Autodesk Inventor part; units mm, degrees
ref_plane "Work Plane1" through (0, 0, 0) normal (0, 0, 1) x (1, 0, 0)
ref_plane "YZ Plane" through (0, 0, 0) normal (1, 0, 0) x (0, 1, 0)
ref_plane "XZ Plane" through (0, 0, 0) normal (0, 1, 0) x (-1, 0, 0)
ref_plane "Work Plane1" through (0, 0, 0) normal (0, 0, 1) x (1, 0, 0)
sketch "Sketch1" plane through (0, 0, 0) normal (0, 0, 1) x (1, 0, 0)
  line L0 (-155.0476, 232.0666) -> (-62.9335, 193.9117) construction
  line L1 (177.2752, 94.414) -> (270.7225, 55.7069) construction
  line L2 (177.2752, -94.414) -> (270.7225, -55.7069) construction
  line L3 (-155.0476, -232.0666) -> (-62.9335, -193.9117) construction
  line L4 (-192.4394, 0.4878) -> (-152.8157, 221.8622) construction
  line L5 (-152.8157, -221.8622) -> (-192.4394, -0.4878) construction
  line L6 (302.4733, 35) -> (302.4733, 38) construction
  line L7 (302.4733, -38) -> (302.4733, -35) construction
  line L8 (-254.8213, 5) -> (-254.8213, -5) construction
  line L9 (-272.5267, 75) -> (-179.1025, 75)
  line L10 (-179.1025, 75) -> (-179.1025, -75)
  line L11 (-179.1025, -75) -> (-272.5267, -75)
  line L12 (-272.5267, -75) -> (-272.5267, 75)
  line L13 (327.4733, 53.8478) -> (327.4733, 38) construction
  line L14 (-272.5267, 5) -> (-272.5267, -5) construction
  line L15 (327.4733, 42.5553) -> (302.4733, 42.5553)
  line L16 (302.4733, 42.5553) -> (302.4733, -42.5553)
  line L17 (302.4733, -42.5553) -> (327.4733, -42.5553)
  line L18 (327.4733, -42.5553) -> (327.4733, 42.5553)
  line L19 (-155.0476, 232.0666) -> (302.4733, 42.5553)
  line L20 (-155.0476, -232.0666) -> (302.4733, -42.5553)
  line L21 (-155.0476, 232.0666) -> (-179.1025, 75)
  line L22 (-179.1025, -75) -> (-155.0476, -232.0666)
  point P0 (0, 0)
  point P1 (-151.2693, 230.5016)
  point P2 (-151.2693, -230.5016)
  dimension "d0" = 150
extrude "Extrusion1" add sketch "Sketch1" along normal blind 10
properties part number "internalSupportBottom1" material "Wood (Birch)"
Could you check a few things on this model? Use its own coordinates, in mm. Coordinates: 2 decimals unless noted, no trailing zeros. Loops run counter-clockwise (first coordinate to the right, second up) from the corner with the lowest first, then second, coordinate; pieces in that order, holes last.
1. I need wall thicknesses on L1, parallel to Y at x = -187.5, z = 0.75; L2, parallel to X at y = 60, z = 3; L3, parallel to Y at x = -125.5, z = 6.5. Which ranges of each line are inside material? Lowest first, please.
2. Imagine slicing it at A-A (z = 4.5). Please give me the cut outline in (x, y), and give its area (3 significant figures).
3. Imagine slicing it at B-B (x = -212). Please give me the cut outline in (y, z).
4. Imagine slicing it at C-C (y = -91.5). Please give me the cut outline in (x, z).
5. For P1, Ø5, axis at x = 121.5, z = 4, coming from the +Y side; P2, Ø1.5, axis at x = -151.5, z = 8.5, coming from the +Y side; P3, Ø4, axis at y = -70.5, z = 2.5, coming from the +X side; P4, Ø5, axis at x = 40.5, y = -154.5, coming from the +Z side, each with a flat end and sliding along its axis, tell me the tip position at first contact or that it passes through.
Computed values:
1. L1: y = -75 to 75
1. L2: x = -272.53 to 260.36
1. L3: y = -219.83 to 219.83
2. outline: (-272.53, -75) - (-179.1, -75) - (-155.05, -232.07) - (302.47, -42.56) - (327.47, -42.56) - (327.47, 42.56) - (302.47, 42.56) - (-155.05, 232.07) - (-179.1, 75) - (-272.53, 75) - close
2. area: 149,000 mm2
3. outline: (-75, 0) - (75, 0) - (75, 10) - (-75, 10) - close
4. outline: (-176.58, 0) - (184.31, 0) - (184.31, 10) - (-176.58, 10) - close
5. P1: stops at y = 118.55
5. P2: stops at y = 230.91
5. P3: stops at x = 239.84
5. P4: passes through
